Verification items for the finished model (mm, model axes). A direction names the side the tool comes from. Coordinates: 2 decimals unless noted, no trailing zeros. Order: outer loops, then holes, each group sorted by start corner. A loop starts at its lowest first (then second) coordinate and runs counter-clockwise, first axis right, second up. Notation, with made-up numbers: M -39,36 L -19,36 A16 cw -19,51 Z; hole C 56.25,33 d4. An arc over 180 degrees is marked long. Return JSON: item names as keys, results as strings.
```python
from build123d import *

# Parameters (mm, degrees)
SKETCH1_W           = 82.6
SKETCH1_H           = 325
SKETCH1_R           = 1.75
BOSS_EXTRUDE4_DEPTH = 1.6
BOSS_EXTRUDE5_DEPTH = 2.3


with BuildPart() as part:
    # Sketch1 → Boss-Extrude4 (new body)
    with BuildSketch(Plane.XY):
        with Locations((-52.667971546, -86.514453125)):
            Rectangle(SKETCH1_W, SKETCH1_H)
        with Locations((-90.767971546, 72.785546875)):
            Circle(SKETCH1_R, mode=Mode.SUBTRACT)
        with Locations((-14.567971546, 72.785546875)):
            Circle(SKETCH1_R, mode=Mode.SUBTRACT)
        with Locations((-14.567971546, -245.814453125)):
            Circle(SKETCH1_R, mode=Mode.SUBTRACT)
        with Locations((-90.767971546, -245.814453125)):
            Circle(SKETCH1_R, mode=Mode.SUBTRACT)
        with Locations((-90.767971546, -114.014453125)):
            Circle(SKETCH1_R, mode=Mode.SUBTRACT)
        with Locations((-14.567971546, -114.014453125)):
            Circle(SKETCH1_R, mode=Mode.SUBTRACT)
        with Locations((-90.767971546, 18.785546875)):
            Circle(SKETCH1_R, mode=Mode.SUBTRACT)
        with Locations((-14.567971546, 18.785546875)):
            Circle(SKETCH1_R, mode=Mode.SUBTRACT)
        Polygon((-92.167971546, -214.714453125), (-79.167971546, -201.714453125), (-26.167971546, -201.714453125), (-13.167971546, -214.714453125), (-13.167971546, -242.014453125), (-92.167971546, -242.014453125), align=None, mode=Mode.SUBTRACT)
        Polygon((-92.167971546, -173.914453125), (-79.167971546, -160.914453125), (-26.167971546, -160.914453125), (-13.167971546, -173.914453125), (-13.167971546, -201.214453125), (-92.167971546, -201.214453125), align=None, mode=Mode.SUBTRACT)
        Polygon((-92.167971546, -37.014453125), (-79.167971546, -24.014453125), (-26.167971546, -24.014453125), (-13.167971546, -37.014453125), (-13.167971546, -64.314453125), (-92.167971546, -64.314453125), align=None, mode=Mode.SUBTRACT)
        Polygon((-92.167971546, -133.114453125), (-79.167971546, -120.114453125), (-26.167971546, -120.114453125), (-13.167971546, -133.114453125), (-13.167971546, -160.414453125), (-92.167971546, -160.414453125), align=None, mode=Mode.SUBTRACT)
        Polygon((-92.167971546, -77.814453125), (-79.167971546, -64.814453125), (-26.167971546, -64.814453125), (-13.167971546, -77.814453125), (-13.167971546, -105.114453125), (-92.167971546, -105.114453125), align=None, mode=Mode.SUBTRACT)
        Polygon((-92.167971546, 3.785546875), (-79.167971546, 16.785546875), (-26.167971546, 16.785546875), (-13.167971546, 3.785546875), (-13.167971546, -23.514453125), (-92.167971546, -23.514453125), align=None, mode=Mode.SUBTRACT)
        Polygon((-92.167971546, 59.085546875), (-79.167970879, 72.085546875), (-26.167970879, 72.085546875), (-13.167971546, 59.085546875), (-13.167971546, 31.785546875), (-92.167971546, 31.785546875), align=None, mode=Mode.SUBTRACT)
    extrude(amount=BOSS_EXTRUDE4_DEPTH)

    # Sketch1_8 → Boss-Extrude5 (add)
    with BuildSketch(Plane.XY):
        Polygon((-92.167971546, 31.785546875), (-92.167971546, 59.085546875), (-79.167970879, 72.085546875), (-26.167970879, 72.085546875), (-13.167971546, 59.085546875), (-13.167971546, 31.785546875), align=None)
        Polygon((-92.167971546, -23.514453125), (-92.167971546, 3.785546875), (-79.167971546, 16.785546875), (-26.167971546, 16.785546875), (-13.167971546, 3.785546875), (-13.167971546, -23.514453125), align=None)
        Polygon((-92.167971546, -64.314453125), (-92.167971546, -37.014453125), (-79.167971546, -24.014453125), (-26.167971546, -24.014453125), (-13.167971546, -37.014453125), (-13.167971546, -64.314453125), align=None)
        Polygon((-92.167971546, -105.114453125), (-92.167971546, -77.814453125), (-79.167971546, -64.814453125), (-26.167971546, -64.814453125), (-13.167971546, -77.814453125), (-13.167971546, -105.114453125), align=None)
        Polygon((-92.167971546, -160.414453125), (-92.167971546, -133.114453125), (-79.167971546, -120.114453125), (-26.167971546, -120.114453125), (-13.167971546, -133.114453125), (-13.167971546, -160.414453125), align=None)
        Polygon((-92.167971546, -201.214453125), (-92.167971546, -173.914453125), (-79.167971546, -160.914453125), (-26.167971546, -160.914453125), (-13.167971546, -173.914453125), (-13.167971546, -201.214453125), align=None)
        Polygon((-92.167971546, -242.014453125), (-92.167971546, -214.714453125), (-79.167971546, -201.714453125), (-26.167971546, -201.714453125), (-13.167971546, -214.714453125), (-13.167971546, -242.014453125), align=None)
    extrude(amount=BOSS_EXTRUDE5_DEPTH)


solid = part.part
```
Q1. Draft check along Y on faces 4 (the face through (-85.759, 10.195, 1.945)), 5 (the face through (-52, -222, 2.3)). Enter one of: pulls with the +Y half, pulls with the -Y half, needs draft (parallel to the pull), parting line crosses it, or undercut.
Values:
{"face 4": "undercut", "face 5": "needs draft"}
Q2. Cross-section at B-B, the plane y = -128. Record the boundary of the cut face in (x, z).
Values:
{"outline": "M -93.97,0 L -11.37,0 L -11.37,1.6 L -18.28,1.6 L -18.28,2.3 L -87.05,2.3 L -87.05,1.6 L -93.97,1.6 Z"}
Q3. Go/stop test with flat-tipped pins: pin 1 (0.6 mm diameter, centred on y = -231.5, z = 2, fed in from +X); pin 2 (6 mm diameter, centred on x = -58.5, y = -64.5, fed in from +Z); pin 3 (0.6 mm diameter, centred on x = -64.5, z = 2, fed in from -Y); pin 4 (0.6 mm diameter, centred on y = -142, z = 2, fed in from -X). Record where each tip stops, or that it passes through.
Values:
{"pin 1": "x = -13.17", "pin 2": "z = 2.3", "pin 3": "y = -242.01", "pin 4": "x = -92.17"}
Q4. Material ranges on line 1 along Z through (x, y) = (-85, 26); line 2 along X through (y, z) = (5.5, 1.9); line 3 along X through (y, z) = (-71.5, 1.9), recorded low to high.
Values:
{"line 1": "0 to 1.6", "line 2": "-90.45 to -14.88", "line 3": "-85.85 to -19.48"}
Q5. Tool access check on faces 1 (the face through (-85.759, -208.305, 1.945)), 2 (the face through (-52, -181, 2.3)), 3 (the face through (-19.76, -167.32, 1.95)). Record the directions out of +Z, -Z, +X, -X, +Y, -Y that give a thin tool (end or side, any length) a straight path to the whole face; none if there is none.
Values:
{"face 1": "+Z, -X", "face 2": "+Z, +X, -X, +Y, -Y", "face 3": "+Z, +X"}
